```python
from build123d import *

# Parameters (mm, degrees)
BOSS_EXTRUDE1_DEPTH = 120
SKETCH4_R           = 3.3
CUT_EXTRUDE1_DEPTH  = 201.688813839
SKETCH5_R           = 2.75
CUT_EXTRUDE2_DEPTH  = 202.285866369
FILLET1_R           = 5


with BuildPart() as part:
    # Sketch2 → Boss-Extrude1 (new body)
    with BuildSketch(Plane.XY):
        Polygon((0, 0), (0, 100), (4, 100), (4, 4), (130, 4), (130, 0), align=None)
    extrude(amount=BOSS_EXTRUDE1_DEPTH)

    # Sketch4 → Cut-Extrude1 (cut, through all)
    with BuildSketch(Plane(origin=(4, 0, 0), x_dir=(0, 0, -1), z_dir=(1, 0, 0))):
        with Locations(Location((-100, 80, 0), (0, 0, 90))):
            Circle(SKETCH4_R)
        with Locations(Location((-20, 80, 0), (0, 0, 90))):
            Circle(SKETCH4_R)
        with Locations(Location((-20, 20, 0), (0, 0, 90))):
            Circle(SKETCH4_R)
        with Locations(Location((-100, 20, 0), (0, 0, 90))):
            Circle(SKETCH4_R)
    extrude(amount=-CUT_EXTRUDE1_DEPTH, mode=Mode.SUBTRACT)

    # Sketch5 → Cut-Extrude2 (cut, through all)
    with BuildSketch(Plane(origin=(0, 4, 0), x_dir=(1, 0, 0), z_dir=(0, 1, 0))):
        with Locations(Location((100, -30, 0), (0, 0, 180))):
            Circle(SKETCH5_R)
        with Locations(Location((50, -30, 0), (0, 0, 180))):
            Circle(SKETCH5_R)
        with Locations(Location((50, -90, 0), (0, 0, 180))):
            Circle(SKETCH5_R)
        with Locations(Location((100, -90, 0), (0, 0, 180))):
            Circle(SKETCH5_R)
    extrude(amount=-CUT_EXTRUDE2_DEPTH, mode=Mode.SUBTRACT)

    # Fillet1
    fillet1_edges = [part.edges().sort_by_distance(p)[0] for p in [
        (4, 4, 60),
    ]]
    fillet(fillet1_edges, radius=FILLET1_R)


solid = part.part
```
The listing builds one solid part. Answer for the finished solid, in the listing's coordinates (mm). Coordinates: 2 decimals unless noted, no trailing zeros. Loops run counter-clockwise (first coordinate to the right, second up) from the corner with the lowest first, then second, coordinate; pieces in that order, holes last. Notation, with made-up numbers: (-38, 44) - (-19, 44) arc R15 ccw to (-19, 54) - close; hole circle Ø6 at (-7.5, -31.5). An arc over 180 degrees is marked (long way). Use a Markdown table: item, result. Add a question column.
1) Given pin 1 (3.5 mm diameter, centred on x = 50, z = 90, fed in from +Y); pin 2 (8 mm diameter, centred on x = 51.5, z = 79.5, fed in from +Y); pin 3 (2 mm diameter, centred on y = 22.5, z = 35.5, fed in from +X), each flat-ended and moving along its own axis, determine where each tip first touches the part or whether it passes through.
2) The part is cut by section C-C, the plane y = 60. Give the vertices of the cut face in (x, z), and give its area (3 significant figures).
3) Find the intervals of material crossed by line 1 (Z direction, x = 100, y = 1); line 2 (Z direction, x = 2.5, y = 80); line 3 (X direction, y = 64, z = 71.5), in increasing order.
4) The part is cut by section A-A, the plane x = 50. Give the vertices of the cut face in (y, z), and give its area (3 significant figures).
5) The mould has two halves that part along Y. Classify faces 1 (the cylindrical face through (2, 76.7, 20.1)), 2 (the cylindrical face through (2.028, 21.774, 102.783)), 3 (the flat face through (4, 55, 59)), 4 (the flat face through (69, 4, 59)): released by +Y, released by -Y, zero draft, split by the parting line, or undercut.
6) The part is cut by section B-B, the plane z = 44. Give the vertices of the cut face in (x, y).
Here are the results:
| question | item | result |
|---|---|---|
| 1 | pin 1 | passes through |
| 1 | pin 2 | stops at y = 4 |
| 1 | pin 3 | stops at x = 4 |
| 2 | outline | (0, 0) - (4, 0) - (4, 120) - (0, 120) - close |
| 2 | area | 480 mm^2 |
| 3 | line 1 | z = 0 to 27.25, 32.75 to 87.25, 92.75 to 120 |
| 3 | line 2 | z = 0 to 16.7, 23.3 to 96.7, 103.3 to 120 |
| 3 | line 3 | x = 0 to 4 |
| 4 | outline | (0, 0) - (4, 0) - (4, 27.25) - (0, 27.25) - close; (0, 32.75) - (4, 32.75) - (4, 87.25) - (0, 87.25) - close; (0, 92.75) - (4, 92.75) - (4, 120) - (0, 120) - close |
| 4 | area | 436 mm^2 |
| 5 | face 1 | undercut |
| 5 | face 2 | undercut |
| 5 | face 3 | zero draft |
| 5 | face 4 | released by +Y |
| 6 | outline | (0, 0) - (130, 0) - (130, 4) - (9, 4) arc R5 cw to (4, 9) - (4, 100) - (0, 100) - close |
